The listing builds one solid part. Answer for the finished solid, in the listing's coordinates (mm). A direction names the side the tool comes from. Coordinates: 2 decimals unless noted, no trailing zeros. Loops run counter-clockwise (first coordinate to the right, second up) from the corner with the lowest first, then second, coordinate; pieces in that order, holes last. Notation, with made-up numbers: (62, 7) - (94, 7) arc R18 cw to (94, 20) - close; hole circle Ø7 at (56, 42.25). An arc over 180 degrees is marked (long way). Return JSON: item names as keys, results as strings. Group by question number.
1. Which of the six approach directions +Z, -Z, +X, -X, +Y, -Y give full straight-line access (tool end or side, diameter ignored) to faces 4 (the face through (-96.22, -0.032, 0.775)), 5 (the face through (-47.7, 0.1, -2.5)), 6 (the face through (-46, 0, 6.5))?
2. Section B-B (x = -77) is taken. Write down the section's boundary in (y, z), and give its area (3 significant figures).
3. Section C-C (z = 3.75) is taken. Write down the section's boundary in (x, y), and give its area (3 significant figures).
4. Section A-A (y = 0) is taken. Write down the section's boundary in (x, z) (3 decimals), and give its area (3 significant figures).
5. Each of these flat-tipped pins is pushed along its axis until it touches: P1, Ø1.4, axis at x = -29.5, y = 0.5, coming from the -Z side; P2, Ø3, axis at y = 0.5, z = -1.5, coming from the +X side; P3, Ø1, axis at y = 0.5, z = 1, coming from the -X side; P4, Ø6.5, axis at x = -100, z = 3.75, coming from the -Y side. Where does it stop, or does it pass through?
6. The mould has two halves that part along X. Classify faces 1 (the face through (-104, -0.03, 3.64)), 2 (the face through (-46, 0, 10)), 3 (the face through (0, 0, 0)): pulls with the +X half, pulls with the -X half, needs draft (parallel to the pull), parting line crosses it, or undercut.
7. Find the intervals of material crossed by line 1 along Y through (x, z) = (-45.5, 8.5); line 2 along Z through (x, y) = (-61, -1.35); line 3 along Z through (x, y) = (-100, 0.05), in increasing order.
```python
from build123d import *


with BuildPart() as part:
    # Sweep1: sweep along a path in Path
    with BuildLine(Plane(origin=(0, 0, 0), x_dir=(1, 0, 0), z_dir=(0, 1, 0))) as sweep1_path:
        Line((0, 0), (-94.005210596, 0))
        ThreePointArc((-94.005210596, 0), (-96.046452048, 0.210549896), (-98.001736865, 0.833333333))
        ThreePointArc((-98.001736865, 0.833333333), (-105, -3.75), (-98.001736865, -8.333333333))
        ThreePointArc((-98.001736865, -8.333333333), (-96.046452048, -7.710549896), (-94.005210596, -7.5))
        Line((-94.005210596, -7.5), (0, -7.5))
    # Cross-section → Sweep1 (sweep)
    with BuildSketch(Plane(origin=(0, 0, 0), x_dir=(0, 0, -1), z_dir=(1, 0, 0))):
        with BuildLine():
            Line((-1, 2.291287847), (-1, -2.291287847))
            ThreePointArc((-1, -2.291287847), (2.5, 0), (-1, 2.291287847))
        make_face()
    sweep(path=sweep1_path.line)


solid = part.part
```
The answers:
{
 "1": {"face 4": "+Y, -Y", "face 5": "+X", "face 6": "+X, +Y, -Y"},
 "2": {"outline": "(-2.29, 1) arc R2.5 ccw (long way) to (2.29, 1) - close; (-2.29, 6.5) - (2.29, 6.5) arc R2.5 ccw (long way) to start", "area": "29.4 mm2"},
 "3": {"outline": "(-104, -2.29) - (-104, 2.29) arc R2.5 ccw (long way) to start", "area": "14.7 mm2"},
 "4": {"outline": "(-98.401, 0.083) arc R4 cw (long way) to (-98.401, 7.417) arc R11 ccw to (-94.005, 6.5) - (0, 6.5) - (0, 10) - (-94.005, 10) arc R7.5 cw to (-97.003, 10.625) arc R7.5 ccw (long way) to (-97.003, -3.125) arc R7.5 cw to (-94.005, -2.5) - (0, -2.5) - (0, 1) - (-94.005, 1) arc R11 ccw to start", "area": "764 mm2"},
 "5": {"P1": "stops at z = -2.5", "P2": "stops at x = 0", "P3": "stops at x = -107.12", "P4": "passes through"},
 "6": {"face 1": "undercut", "face 2": "needs draft", "face 3": "pulls with the +X half"},
 "7": {"line 1": "y = -2.29 to 2.29", "line 2": "z = -2.1 to 1, 6.5 to 9.6", "line 3": "z = -3.75 to -0.25, 7.75 to 11.25"}
}
